from build123d import *

# Parameters (mm, degrees)
F2_R     = 1.5
F3_R     = 2
F4_DEPTH = 25
F5_W     = 3
F5_H     = 5
F6_DEPTH = 50


with BuildPart() as f1:
    # F0 (on Front) → F1 (revolve)
    with BuildSketch(Plane.XZ):
        Polygon((8.911915, -3), (-14.088085, -3), (-14.088085, -7), (1.911915, -7), (1.911915, -14), (-4.088085, -14), (-4.088085, -22), (-0.088085, -22), (-0.088085, -18), (8.911915, -18), (8.911915, -22), (12.911915, -22), (12.911915, -14), (5.911915, -14), (5.911915, -7), (8.911915, -7), align=None)
    revolve(axis=Axis((-1.3057, 0, 0), (1, 0, 0)))

    # F2
    f2_edges = [f1.edges().sort_by_distance(p)[0] for p in [
        (1.911915, 0, 7),
        (1.911915, 0, 14),
    ]]
    fillet(f2_edges, radius=F2_R)

    # F3 (on face) → F4 (cut)
    with BuildSketch(Plane(origin=(1.911915, 0, 0), x_dir=(0, -1, 0), z_dir=(-1, 0, 0))):
        with Locations((-10.5, 0)):
            Circle(F3_R)
        with Locations((-7.424621, -7.424621)):
            Circle(F3_R)
        with Locations((0, -10.5)):
            Circle(F3_R)
        with Locations((7.424621, -7.424621)):
            Circle(F3_R)
        with Locations((10.5, 0)):
            Circle(F3_R)
        with Locations((7.424621, 7.424621)):
            Circle(F3_R)
        with Locations((0, 10.5)):
            Circle(F3_R)
        with Locations((-7.424621, 7.424621)):
            Circle(F3_R)
    extrude(amount=-F4_DEPTH, mode=Mode.SUBTRACT)

    # F5 (on face) → F6 (cut)
    with BuildSketch(Plane(origin=(-14.088085, 0, 0), x_dir=(0, -1, 0), z_dir=(-1, 0, 0))):
        with Locations((0.026283, 2.5)):
            Rectangle(F5_W, F5_H)
    extrude(amount=-F6_DEPTH, mode=Mode.SUBTRACT)


solid = f1.part
Could you check a few things on this model? Use its own coordinates, in mm. A direction names the side the tool comes from. Round coordinates to 2 decimals unless told otherwise and drop trailing zeros. Order: outer loops, then holes, each group sorted by start corner. A loop starts at its lowest first (then second) coordinate and runs counter-clockwise, first axis right, second up.
Q1. Imagine slicing it at A-A, the plane x = -5. List the corners of the cut face in (y, z) for me.
Geometry says:
outline: circle Ø14 at (0, 0); hole (-1.53, 2.58) arc R3 ccw (long way) to (1.47, 2.61) - (1.47, 5) - (-1.53, 5) - close
Q2. I'm going to push flat-ended pins straight in: P1, Ø1, axis at y = 16.5, z = -11, coming from the -X side; P2, Ø22.5, axis at y = 2, z = 5.5, coming from the +X side; P3, Ø5, axis at y = -10.5, z = 0, coming from the -X side; P4, Ø4, axis at x = 3, y = 5.5, coming from the -Z side. Where does each tip first touch, or does it pass through?
Geometry says:
P1: stops at x = -4.09
P2: stops at x = 12.91
P3: stops at x = 1.83
P4: stops at z = -17.66
Q3. Please list where these lines run through material, in increasing order: probe 1 along Z at (x, y) = (6, 0.5); probe 2 along X at (y, z) = (-18, -11); probe 3 along X at (y, z) = (-6, -1.5).
Geometry says:
probe 1: z = -17.99 to -13.99, -6.98 to -2.96, 5 to 6.98, 13.99 to 17.99
probe 2: x = -4.09 to -0.09, 8.91 to 12.91
probe 3: x = -14.09 to 8.91
Q4. Thinking about a two-plate mould opening in Z: for faces 1 (the face through (4.475, 17.847, 2.343)), 2 (the face through (-4.088, 0.3, 14.4)), 3 (the face through (-1.87, -5.362, -12.932)), 4 (the face through (3.9, -8.9, -1.2)), which applies, released by +Z, released by -Z, zero draft, split by the parting line, or undercut?
Geometry says:
face 1: split by the parting line
face 2: zero draft
face 3: undercut
face 4: undercut
Q5. Imagine slicing it at B-B, the plane y = -16. List the corners of the cut face in (x, z) for me.
Geometry says:
outline: (-4.09, -15.1) - (-0.09, -15.1) - (-0.09, -8.25) - (8.91, -8.25) - (8.91, -15.1) - (12.91, -15.1) - (12.91, 15.1) - (8.91, 15.1) - (8.91, 8.25) - (-0.09, 8.25) - (-0.09, 15.1) - (-4.09, 15.1) - close
Q6. Which directions (+Z, -Z, +X, -X, +Y, -Y) give clear straight access to the entire face, cutting with the end or side of a thin tool? Please do faces 5 (the face through (1.912, 4, -10)), 6 (the face through (8.912, -16.2, -8.3)), 7 (the face through (-3, -1.526, 4)).
Geometry says:
face 5: -X
face 6: none
face 7: +X, -X
